Here's how the part is built. I have some questions about the finished solid (model axes, mm). Give positions to 0.01 mm unless a question says otherwise; leave off trailing zeros. Loops run counter-clockwise (first coordinate to the right, second up) from the corner with the lowest first, then second, coordinate; pieces in that order, holes last.
Q1. I need wall thicknesses on line 1 (Y direction, x = 0, z = 1.9); line 2 (X direction, y = -1.5, z = 2.65); line 3 (X direction, y = 24, z = 1.55). Which ranges of each line are inside material? Lowest first, please.
Q2. If we section it at A-A (x = 0): Please give me the cut outline in (y, z), plus the area to 3 significant figures.
Q3. If we section it at C-C (x = -42.5): Please give me the cut outline in (y, z).
Q4. If we section it at D-D (z = 2.85): Give the number of separate pieces and of enclosed holes in the cut face, plus the area to 3 significant figures.
Q5. If we section it at B-B (y = 16.5): Please give me the cut outline in (x, z), plus the area to 3 significant figures.
Q6. Will these pins go through, and if not, where does the flat tip stop? P1, Ø5, axis at x = -30.05, y = 22.96, coming from the +Z side; P2, Ø1, axis at x = 4, z = 2, coming from the +Y side; P3, Ø0.8, axis at y = 6, z = 2.5, coming from the +X side; P4, Ø1, axis at y = 6.5, z = 2, coming from the -X side.
from build123d import *

# Parameters (mm, degrees)
SKETCH_3_R      = 1.5
SKETCH_3_R_2    = 2
EXTRUDE_1_DEPTH = 4


with BuildPart() as part:
    # 草图3 → 凸台-拉伸1 (new body)
    with BuildSketch(Plane.XY):
        with BuildLine():
            Line((-46.5, -7.990216685), (46.5, -7.990216685))
            Line((46.5, -7.990216685), (46.5, 0.009783315))
            Line((46.5, 0.009783315), (49.5, 0.009783315))
            Line((49.5, 0.009783315), (49.5, 5.009783315))
            Line((49.5, 5.009783315), (46.5, 5.009783315))
            Line((46.5, 5.009783315), (46.5, 7.009783315))
            Line((46.5, 7.009783315), (44, 7.009783315))
            Line((44, 7.009783315), (44, 5.509783315))
            Line((44, 5.509783315), (41.4, 5.509783315))
            Line((41.4, 5.509783315), (41.4, 7.009783315))
            Line((41.4, 7.009783315), (38.4, 7.009783315))
            Line((38.4, 7.009783315), (38.4, 10.009783315))
            Line((38.4, 10.009783315), (41.4, 10.009783315))
            Line((41.4, 10.009783315), (41.4, 11.509783315))
            Line((41.4, 11.509783315), (44, 11.509783315))
            Line((44, 11.509783315), (44, 10.009783315))
            Line((44, 10.009783315), (46.5, 10.009783315))
            Line((46.5, 10.009783315), (46.5, 15.009783315))
            Line((46.5, 15.009783315), (49.5, 15.009783315))
            Line((49.5, 15.009783315), (49.5, 20.009783315))
            Line((49.5, 20.009783315), (46.5, 20.009783315))
            Line((46.5, 20.009783315), (46.5, 30.009783315))
            Line((46.5, 30.009783315), (34.06116735, 36.162324196))
            ThreePointArc((34.06116735, 36.162324196), (-11.38853896, 16.756491321), (-37.576612526, 58.666477673))
            Line((-37.576612526, 58.666477673), (-46.5, 60.009783315))
            Line((-46.5, 60.009783315), (-46.5, 20.009783315))
            Line((-46.5, 20.009783315), (-49.5, 20.009783315))
            Line((-49.5, 20.009783315), (-49.5, 15.009783315))
            Line((-49.5, 15.009783315), (-46.5, 15.009783315))
            Line((-46.5, 15.009783315), (-46.5, 10.009783315))
            Line((-46.5, 10.009783315), (-44, 10.009783315))
            Line((-44, 10.009783315), (-44, 11.509783315))
            Line((-44, 11.509783315), (-41.4, 11.509783315))
            Line((-41.4, 11.509783315), (-41.4, 10.009783315))
            Line((-41.4, 10.009783315), (-38.4, 10.009783315))
            Line((-38.4, 10.009783315), (-38.4, 7.009783315))
            Line((-38.4, 7.009783315), (-41.4, 7.009783315))
            Line((-41.4, 7.009783315), (-41.4, 5.509783315))
            Line((-41.4, 5.509783315), (-44, 5.509783315))
            Line((-44, 5.509783315), (-44, 7.009783315))
            Line((-44, 7.009783315), (-46.5, 7.009783315))
            Line((-46.5, 7.009783315), (-46.5, 5.009783315))
            Line((-46.5, 5.009783315), (-49.5, 5.009783315))
            Line((-49.5, 5.009783315), (-49.5, 0.009783315))
            Line((-49.5, 0.009783315), (-46.5, 0.009783315))
            Line((-46.5, 0.009783315), (-46.5, -7.990216685))
        make_face()
        with Locations((-31.5, -0.990216685)):
            Circle(SKETCH_3_R, mode=Mode.SUBTRACT)
        with Locations((31.5, -0.990216685)):
            Circle(SKETCH_3_R, mode=Mode.SUBTRACT)
        with Locations((0, 10.509783315)):
            Circle(SKETCH_3_R_2, mode=Mode.SUBTRACT)
        with Locations((-30.0520382, 22.957745114)):
            Circle(SKETCH_3_R_2, mode=Mode.SUBTRACT)
        with Locations((-42.5, 53.009783315)):
            Circle(SKETCH_3_R_2, mode=Mode.SUBTRACT)
        with Locations((30.0520382, 22.957745114)):
            Circle(SKETCH_3_R_2, mode=Mode.SUBTRACT)
    extrude(amount=EXTRUDE_1_DEPTH)


solid = part.part
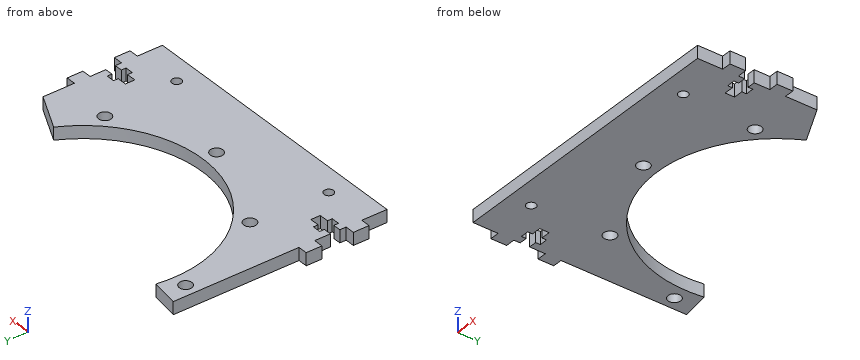
Check sheet entries:
1. line 1: y = -7.99 to 8.51, 12.51 to 15.01
1. line 2: x = -46.5 to -32.91, -30.09 to 30.09, 32.91 to 46.5
1. line 3: x = -46.5 to -31.76, -28.35 to -24.54, 24.54 to 28.35, 31.76 to 46.5
2. outline: (-7.99, 0) - (8.51, 0) - (8.51, 4) - (-7.99, 4) - close; (12.51, 0) - (15.01, 0) - (15.01, 4) - (12.51, 4) - close
2. area: 76.0 mm2
3. outline: (-7.99, 0) - (5.51, 0) - (5.51, 4) - (-7.99, 4) - close; (11.51, 0) - (51.01, 0) - (51.01, 4) - (11.51, 4) - close; (55.01, 0) - (59.41, 0) - (59.41, 4) - (55.01, 4) - close
4. separate pieces: 1
4. enclosed holes: 6
4. area: 3,190 mm2
5. outline: (-49.5, 0) - (-10.54, 0) - (-10.54, 4) - (-49.5, 4) - close; (10.54, 0) - (49.5, 0) - (49.5, 4) - (10.54, 4) - close
5. area: 312 mm2
6. P1: stops at z = 4
6. P2: stops at y = 15.28
6. P3: stops at x = 46.5
6. P4: stops at x = -46.5
